Design review of the part shown in the three views and the two pictorial views. Dimensions are in mm from the part's minimum x, y and z. Give positions to 0.01 mm unless a question says otherwise; leave off trailing zeros. Loops run counter-clockwise (first coordinate to the right, second up) from the corner with the lowest first, then second, coordinate; pieces in that order, holes last. Notation, with made-up numbers: (48.25, 64) - (81.25, 64) arc R13 cw to (81.25, 75) - close; hole circle Ø3 at (-23.75, 10.25). An arc over 180 degrees is marked (long way). Put each result on its own line as item: value. Start each with the question number.
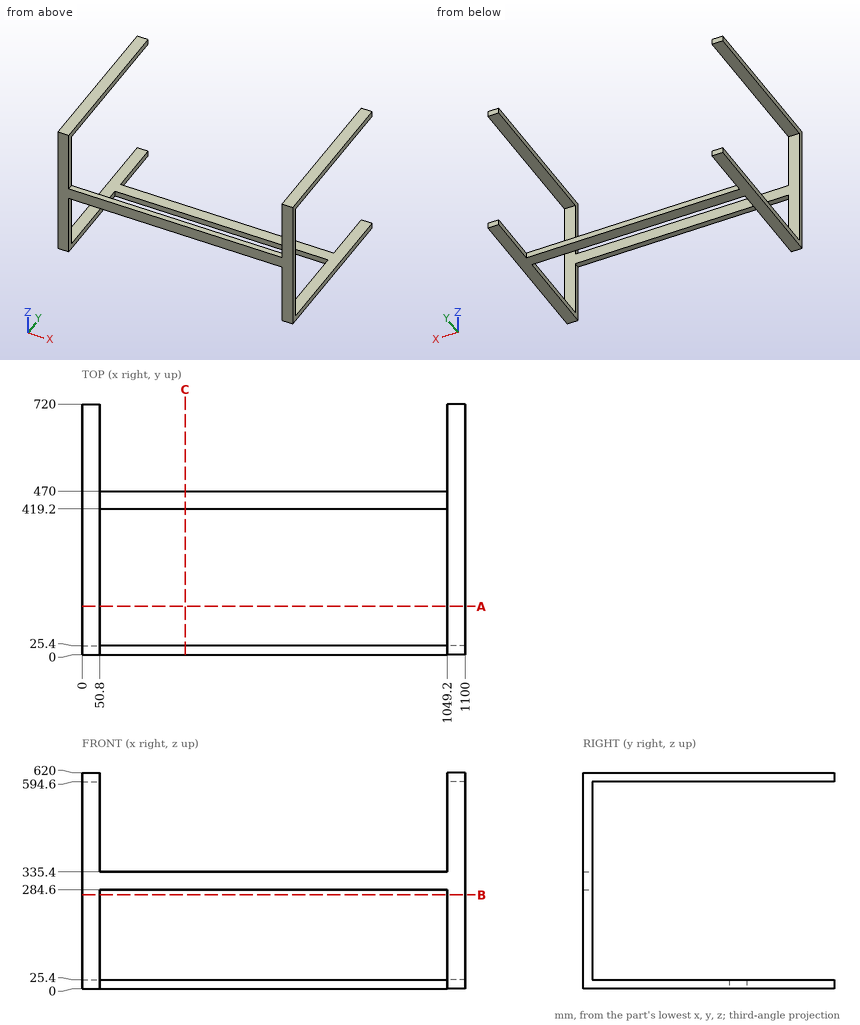
1) Insertion check: P1, Ø7.5, axis at x = 307, y = 10, coming from the +Z side; P2, Ø12.5, axis at x = 319.5, y = 11.5, coming from the -Z side; P3, Ø12.5, axis at x = 379, z = 10, coming from the +Y side. Each pin has a flat end and moves straight along its axis. Give the tip position at first contact, or say it passes through.
2) Wall thickness on probe 1 along Y at (x, z) = (613, 305): over which ranges is the line inside the solid? List them lowest first.
3) Take a section at B-B on z = 269.5. State the section outline as (x, y) points, and give its area (3 significant figures).
4) Take a section at C-C on x = 296. State the section outline as (y, z) points, and give its area (3 significant figures).
5) Take a section at A-A on y = 139. State the section outline as (x, z) points.
Answers follow:
1. P1: z = 335.4
1. P2: z = 284.6
1. P3: y = 470
2. probe 1: 0 to 25.4
3. outline: (0, 0) - (50.8, 0) - (50.8, 25.4) - (0, 25.4) - close; (1049.2, 0) - (1100, 0) - (1100, 25.4) - (1049.2, 25.4) - close
3. area: 2,580 mm2
4. outline: (0, 284.6) - (25.4, 284.6) - (25.4, 335.4) - (0, 335.4) - close; (419.2, 0) - (470, 0) - (470, 25.4) - (419.2, 25.4) - close
4. area: 2,580 mm2
5. outline: (0, 0) - (50.8, 0) - (50.8, 25.4) - (0, 25.4) - close; (0, 594.6) - (50.8, 594.6) - (50.8, 620) - (0, 620) - close; (1049.2, 0) - (1100, 0) - (1100, 25.4) - (1049.2, 25.4) - close; (1049.2, 594.6) - (1100, 594.6) - (1100, 620) - (1049.2, 620) - close
